Input: part model. Units: mm. Frame: model coordinates. A direction names the side the tool comes from. Give positions to 0.01 mm unless a question says otherwise; leave off trailing zeros. Loops run counter-clockwise (first coordinate to the right, second up) from the corner with the lowest first, then second, coordinate; pieces in that order, holes last. Notation, with made-up numbers: (75.25, -13) -> (131.25, -13) arc R25 ccw to (131.25, 19) -> close; hole circle Ø7 at (40, 86.25). An arc over 180 degrees is marked (long way). Use CSV: the item, a comma, the result in double quotes.
```python
from build123d import *

# Parameters (mm, degrees)
SKETCH1_W           = 44.45
SKETCH1_H           = 19.05
BOSS_EXTRUDE1_DEPTH = 6.985
BOSS_EXTRUDE3_START = 1.5875
SKETCH4_R           = 1.5
BOSS_EXTRUDE3_DEPTH = 2.54
SKETCH5_R           = 5.08
BOSS_EXTRUDE4_DEPTH = 2.286
FILLET3_R           = 2.54
FILLET4_R           = 2.54
SKETCH7_W           = 31.75
SKETCH7_H           = 15.875
CUT_EXTRUDE1_DEPTH  = 4.445
SKETCH8_W           = 38.354
SKETCH8_H           = 15.875
CUT_EXTRUDE2_DEPTH  = 1.9558
BOSS_EXTRUDE5_DEPTH = 2.54
FILLET5_R           = 2.54
SKETCH12_R          = 1.4
CUT_EXTRUDE5_DEPTH  = 6.985


with BuildPart() as part:
    # Sketch1 → Boss-Extrude1 (new body)
    with BuildSketch(Plane.XY):
        Rectangle(SKETCH1_W, SKETCH1_H)
    extrude(amount=BOSS_EXTRUDE1_DEPTH)

    # Sketch4 → Boss-Extrude3 (add)
    with BuildSketch(Plane(origin=(0, 0, 0), x_dir=(0, 0, -1), z_dir=(1, 0, 0)).offset(BOSS_EXTRUDE3_START)):
        with BuildLine():
            Line((0, 9.525), (6.35, 9.525))
            ThreePointArc((6.35, 9.525), (11.43, 4.445), (6.35, -0.635))
            Line((6.35, -0.635), (0, -0.635))
            Line((0, -0.635), (0, 9.525))
        make_face()
        with Locations((6.35, 4.445)):
            Circle(SKETCH4_R, mode=Mode.SUBTRACT)
    boss_extrude3 = extrude(amount=BOSS_EXTRUDE3_DEPTH)

    # Mirror1: Boss-Extrude3 across plane
    add(boss_extrude3.mirror(Plane(origin=(0, 0, 0), x_dir=(0, 0, 1), z_dir=(1, 0, 0))))

    # Sketch5 → Boss-Extrude4 (add)
    with BuildSketch(Plane(origin=(4.1275, 0, 0), x_dir=(0, 0, -1), z_dir=(1, 0, 0))):
        with Locations(Location((6.35, 4.445, 0), (0, 0, 90))):
            Circle(SKETCH5_R)
        Polygon((8.183087105, 7.62), (4.516912895, 7.62), (2.683825791, 4.445), (4.516912895, 1.27), (8.183087105, 1.27), (10.016174209, 4.445), align=None, mode=Mode.SUBTRACT)
    extrude(amount=BOSS_EXTRUDE4_DEPTH)

    # Fillet3
    # the kernel refuses this fillet: 2.54 mm, written as the material it adds along each edge
    with BuildSketch(Plane(origin=(-4.1275, -0.635, 0), x_dir=(-1, 0, 0), z_dir=(0, 1, 0))) as fillet3_piece_1:
        with BuildLine():
            CenterArc((FILLET3_R, -FILLET3_R), FILLET3_R, 90, 90)
            Line((0, -FILLET3_R), (0, 0))
            Line((0, 0), (FILLET3_R, 0))
        make_face()
    extrude(amount=10.16)
    with BuildSketch(Plane(origin=(4.1275, -0.635, 0), x_dir=(1, 0, 0), z_dir=(0, 1, 0))) as fillet3_piece_2:
        with BuildLine():
            CenterArc((FILLET3_R, FILLET3_R), FILLET3_R, 180, 90)
            Line((0, FILLET3_R), (0, 0))
            Line((0, 0), (FILLET3_R, 0))
        make_face()
    extrude(amount=10.16)

    # Fillet4
    fillet4_edges = [part.edges().sort_by_distance(p)[0] for p in [
        (-4.1275, -0.635, 0),
        (4.1275, -0.635, 0),
    ]]
    fillet(fillet4_edges, radius=FILLET4_R)

    # Sketch7 → Cut-Extrude1 (cut)
    with BuildSketch(Plane.XY.offset(6.985)):
        with Locations((0, 1.5875)):
            Rectangle(SKETCH7_W, SKETCH7_H)
    extrude(amount=-CUT_EXTRUDE1_DEPTH, mode=Mode.SUBTRACT)

    # Sketch8 → Cut-Extrude2 (cut)
    with BuildSketch(Plane.XY.offset(6.985)):
        with Locations((0, 1.5875)):
            Rectangle(SKETCH8_W, SKETCH8_H)
    extrude(amount=-CUT_EXTRUDE2_DEPTH, mode=Mode.SUBTRACT)

    # Sketch9 → Boss-Extrude5 (add)
    with BuildSketch(Plane.XY.offset(6.985)):
        Polygon((-22.225, 9.525), (-15.875, 9.525), (-15.875, -6.35), (15.875, -6.35), (15.875, 9.525), (22.225, 9.525), (22.225, -9.525), (-22.225, -9.525), align=None)
    extrude(amount=BOSS_EXTRUDE5_DEPTH)

    # Fillet5
    fillet5_edges = [part.edges().sort_by_distance(p)[0] for p in [
        (22.225, -9.525, 4.7625),
        (-22.225, -9.525, 4.7625),
    ]]
    fillet(fillet5_edges, radius=FILLET5_R)

    # Sketch12 → Cut-Extrude5 (cut)
    with BuildSketch(Plane(origin=(0, 0, 0), x_dir=(-1, 0, 0), z_dir=(0, 0, -1))):
        with Locations((-17.653, -1.905)):
            Circle(SKETCH12_R)
        with Locations((17.653, -1.905)):
            Circle(SKETCH12_R)
    extrude(amount=-CUT_EXTRUDE5_DEPTH, mode=Mode.SUBTRACT)


solid = part.part
```
1) Reachability of faces 1 (the flat face through (-15.875, 2, 8)), 2 (the flat face through (5.254, 2.88, -3.588)), 3 (the flat face through (6.414, 8, -6)) from +Z, -Z, +X, -X, +Y, -Y: full face, straight path, thin tool, end or side. Return the list, or none.
From the geometry:
face 1,"+Z, +Y"
face 2,"+X"
face 3,"-Z, +X, +Y, -Y"
2) Section query C-C (z = 2). Return loops of the section in (x, y) (3 decimals), then the cut area to 3 significant figures.
From the geometry:
outline,"(-22.225, -6.985) arc R2.54 ccw to (-19.685, -9.525) -> (19.685, -9.525) arc R2.54 ccw to (22.225, -6.985) -> (22.225, 9.525) -> (-22.225, 9.525) -> close; hole circle Ø2.8 at (-17.653, -1.905); hole circle Ø2.8 at (17.653, -1.905)"
area,"832 mm^2"
3) Section query D-D (z = -1.75). Return loops of the section in (x, y) (1 decimal).
From the geometry:
outline,"(-4.3, -0.8) -> (-1.6, -0.8) -> (-1.6, 9.5) -> (-4.3, 9.5) -> close; (1.6, -0.8) -> (4.3, -0.8) -> (4.3, 2.3) -> (6.4, 2.3) -> (6.4, 6.6) -> (4.3, 6.6) -> (4.3, 9.5) -> (1.6, 9.5) -> close"
4) Section query A-A (x = 5.5). Give the number of separate pieces and of enclosed holes in the cut face, then the cut area to 3 significant figures.
From the geometry:
separate pieces,"2"
enclosed holes,"1"
area,"120 mm^2"
5) Section query B-B (x = -2.5). Return loops of the section in (y, z) (3 decimals), then the cut area to 3 significant figures.
From the geometry:
outline,"(-9.525, 0) -> (-3.175, 0) arc R2.54 cw to (-0.635, -2.54) -> (-0.635, -6.35) arc R5.08 ccw to (9.525, -6.35) -> (9.525, 2.54) -> (-6.35, 2.54) -> (-6.35, 9.525) -> (-9.525, 9.525) -> close; hole circle Ø3 at (4.445, -6.35)"
area,"170 mm^2"
6) Mould query, pull axis Y, two halves, no side actions, for faces 4 (the cylindrical face through (3.527, -1.741, -0.443)), 5 (the cylindrical face through (-18.946, -2.441, 2.479)), 6 (the flat face through (-15.875, 1, 4)), 7 (the flat face through (5, 7.62, -6)). Classes: pulls with the +Y half, pulls with the -Y half, needs draft (parallel to the pull), parting line crosses it, or undercut.
From the geometry:
face 4,"pulls with the -Y half"
face 5,"undercut"
face 6,"needs draft"
face 7,"undercut"
7) Ray query, line 1 (X direction, y = 0, z = -8.5); line 2 (X direction, y = 4.25, z = -8.25); line 3 (Z direction, x = -14, y = -5.25). Return the intervals inside material, ascending.
From the geometry:
line 1,"x = -4.13 to -1.59, 1.59 to 6.41"
line 2,"x = -4.13 to -1.59, 1.59 to 4.13"
line 3,"z = 0 to 2.54"
8) Contact query for flat-ended pins moving along their axis: pin 1 (8 mm diameter, centred on y = -1.5, z = -4.5, fed in from -X); pin 2 (1.5 mm diameter, centred on x = 12.5, y = -0.5, fed in from -Z); pin 3 (3.5 mm diameter, centred on y = 4.445, z = -6.35, fed in from +X); pin 4 (2.5 mm diameter, centred on y = 4.445, z = -6.35, fed in from +X). Output: stop coordinate, or through.
From the geometry:
pin 1,"stops at x = -5.15"
pin 2,"stops at z = 0"
pin 3,"stops at x = 4.13"
pin 4,"passes through"
